from build123d import *
from OCP.BRepFilletAPI import BRepFilletAPI_MakeChamfer
from build123d.topology import SkipClean

# Parameters (mm, degrees)
SKETCH1_R                 = 12
SKETCH1_R_2               = 8
BOSS_EXTRUDE4_DEPTH       = 2
BOSS_EXTRUDE5_START       = 2
SKETCH1_9_R               = 12
SKETCH1_9_R_2             = 9
BOSS_EXTRUDE5_DEPTH       = 4
BOSS_EXTRUDE6_START       = 2
BOSS_EXTRUDE6_DEPTH       = 2
BOSS_EXTRUDE7_START       = 4
BOSS_EXTRUDE7_DEPTH       = 2
SKETCH1_12_W              = 60
SKETCH1_12_H              = 60
SKETCH1_12_R              = 12
SKETCH1_12_R_2            = 9
SKETCH1_12_R_3            = 8
BOSS_EXTRUDE8_DEPTH       = 2
BOSS_EXTRUDE9_DEPTH       = 6
CHAMFER1_SIZE             = 1
CHAMFER1_SIZE2            = 0.176326981
BOSS_EXTRUDE10_DEPTH      = 6
BOSS_EXTRUDE11_DEPTH      = 20
BOSS_EXTRUDE12_DEPTH      = 2
BOSS_EXTRUDE12_DEPTH_BACK = 2
SKETCH1_14_R              = 8
CUT_EXTRUDE1_DEPTH        = 47.904157598


with BuildPart() as part:
    # Sketch1 → Boss-Extrude4 (new body)
    with BuildSketch(Plane(origin=(0, 0, 0), x_dir=(1, 0, 0), z_dir=(0, 1, 0))):
        with Locations(Location((0, 0, 0), (0, 0, 270))):
            Circle(SKETCH1_R)
        with Locations(Location((0, 0, 0), (0, 0, 270))):
            Circle(SKETCH1_R_2, mode=Mode.SUBTRACT)
    extrude(amount=BOSS_EXTRUDE4_DEPTH)

    # Sketch1<9> → Boss-Extrude5 (add)
    with BuildSketch(Plane(origin=(0, 0, 0), x_dir=(1, 0, 0), z_dir=(0, 1, 0)).offset(BOSS_EXTRUDE5_START)):
        with Locations(Location((0, 0, 0), (0, 0, 270))):
            Circle(SKETCH1_9_R)
        with Locations(Location((0, 0, 0), (0, 0, 270))):
            Circle(SKETCH1_9_R_2, mode=Mode.SUBTRACT)
    extrude(amount=BOSS_EXTRUDE5_DEPTH)

    # Sketch1<10> → Boss-Extrude6 (add)
    with SkipClean():  # the faces are left unmerged after this step: merging them gives an invalid solid
        with BuildSketch(Plane(origin=(0, 0, 0), x_dir=(1, 0, 0), z_dir=(0, 1, 0)).offset(BOSS_EXTRUDE6_START)):
            with BuildLine():
                ThreePointArc((0, 8), (2.070552361, 7.72740661), (4, 6.92820323))
                Line((4, 6.92820323), (4.5, 7.794228634))
                ThreePointArc((4.5, 7.794228634), (2.329371406, 8.693332437), (0, 9))
                Line((0, 9), (0, 8))
            make_face()
            with BuildLine():
                ThreePointArc((-8, 0), (-7.72740661, 2.070552361), (-6.92820323, 4))
                Line((-6.92820323, 4), (-7.794228634, 4.5))
                ThreePointArc((-7.794228634, 4.5), (-8.693332437, 2.329371406), (-9, 0))
                Line((-9, 0), (-8, 0))
            make_face()
            with BuildLine():
                Line((0, -9), (0, -8))
                ThreePointArc((0, -8), (-2.070552361, -7.72740661), (-4, -6.92820323))
                Line((-4, -6.92820323), (-4.5, -7.794228634))
                ThreePointArc((-4.5, -7.794228634), (-2.329371406, -8.693332437), (0, -9))
            make_face()
            with BuildLine():
                Line((9, 0), (8, 0))
                ThreePointArc((8, 0), (7.72740661, -2.070552361), (6.92820323, -4))
                Line((6.92820323, -4), (7.794228634, -4.5))
                ThreePointArc((7.794228634, -4.5), (8.693332437, -2.329371406), (9, 0))
            make_face()
        extrude(amount=BOSS_EXTRUDE6_DEPTH)

    # Sketch1<11> → Boss-Extrude7 (add)
    with SkipClean():  # the faces are left unmerged after this step: merging them gives an invalid solid
        with BuildSketch(Plane(origin=(0, 0, 0), x_dir=(1, 0, 0), z_dir=(0, 1, 0)).offset(BOSS_EXTRUDE7_START)):
            with BuildLine():
                ThreePointArc((0, 8), (2.070552361, 7.72740661), (4, 6.92820323))
                Line((4, 6.92820323), (4.5, 7.794228634))
                ThreePointArc((4.5, 7.794228634), (2.329371406, 8.693332437), (0, 9))
                Line((0, 9), (0, 8))
            make_face()
            with BuildLine():
                ThreePointArc((4, 6.92820323), (5.656854249, 5.656854249), (6.92820323, 4))
                Line((6.92820323, 4), (7.794228634, 4.5))
                ThreePointArc((7.794228634, 4.5), (6.363961031, 6.363961031), (4.5, 7.794228634))
                Line((4.5, 7.794228634), (4, 6.92820323))
            make_face()
            with BuildLine():
                ThreePointArc((-8, 0), (-7.72740661, 2.070552361), (-6.92820323, 4))
                Line((-6.92820323, 4), (-7.794228634, 4.5))
                ThreePointArc((-7.794228634, 4.5), (-8.693332437, 2.329371406), (-9, 0))
                Line((-9, 0), (-8, 0))
            make_face()
            with BuildLine():
                ThreePointArc((-6.92820323, 4), (-5.656854249, 5.656854249), (-4, 6.92820323))
                Line((-4, 6.92820323), (-4.5, 7.794228634))
                ThreePointArc((-4.5, 7.794228634), (-6.363961031, 6.363961031), (-7.794228634, 4.5))
                Line((-7.794228634, 4.5), (-6.92820323, 4))
            make_face()
            with BuildLine():
                Line((-4.5, -7.794228634), (-4, -6.92820323))
                ThreePointArc((-4, -6.92820323), (-5.656854249, -5.656854249), (-6.92820323, -4))
                Line((-6.92820323, -4), (-7.794228634, -4.5))
                ThreePointArc((-7.794228634, -4.5), (-6.363961031, -6.363961031), (-4.5, -7.794228634))
            make_face()
            with BuildLine():
                Line((0, -9), (0, -8))
                ThreePointArc((0, -8), (-2.070552361, -7.72740661), (-4, -6.92820323))
                Line((-4, -6.92820323), (-4.5, -7.794228634))
                ThreePointArc((-4.5, -7.794228634), (-2.329371406, -8.693332437), (0, -9))
            make_face()
            with BuildLine():
                Line((9, 0), (8, 0))
                ThreePointArc((8, 0), (7.72740661, -2.070552361), (6.92820323, -4))
                Line((6.92820323, -4), (7.794228634, -4.5))
                ThreePointArc((7.794228634, -4.5), (8.693332437, -2.329371406), (9, 0))
            make_face()
            with BuildLine():
                Line((7.794228634, -4.5), (6.92820323, -4))
                ThreePointArc((6.92820323, -4), (5.656854249, -5.656854249), (4, -6.92820323))
                Line((4, -6.92820323), (4.5, -7.794228634))
                ThreePointArc((4.5, -7.794228634), (6.363961031, -6.363961031), (7.794228634, -4.5))
            make_face()
        extrude(amount=BOSS_EXTRUDE7_DEPTH)

    # Sketch1<12> → Boss-Extrude8 (add)
    # profile 1 of 2: a face of its own
    with BuildSketch(Plane(origin=(0, 0, 0), x_dir=(1, 0, 0), z_dir=(0, 1, 0))):
        Rectangle(SKETCH1_12_W, SKETCH1_12_H)
        with Locations(Location((0, 0, 0), (0, 0, 270))):
            Circle(SKETCH1_12_R, mode=Mode.SUBTRACT)
    # profile 2 of 2: a face of its own
    with BuildSketch(Plane(origin=(0, 0, 0), x_dir=(1, 0, 0), z_dir=(0, 1, 0))):
        Circle(SKETCH1_12_R_2)
        with Locations(Location((0, 0, 0), (0, 0, 270))):
            Circle(SKETCH1_12_R_3, mode=Mode.SUBTRACT)
    extrude(amount=BOSS_EXTRUDE8_DEPTH)

    # Sketch3 → Boss-Extrude9 (add)
    with BuildSketch(Plane.XZ):
        Polygon((-30, -30), (30, -30), (30, -28), (-28, -28), (-28, 30), (-30, 30), align=None)
        Polygon((30, -26), (30, -24), (-24, -24), (-24, 30), (-26, 30), (-26, -26), align=None)
    extrude(amount=BOSS_EXTRUDE9_DEPTH)

    # Chamfer1: one chamfer whose edges measure the first distance from different faces: ONE call of the kernel's chamfer builder (chamfer() names one face for all edges)
    chamfer1_edges_1 = [part.edges().sort_by_distance(p)[0] for p in [
        (-28, -6, 1),
    ]]
    chamfer1_side_1 = [part.faces().sort_by_distance(p)[0] for p in [
        (-28, -3, 1),
    ]]
    chamfer1_edges_2 = [part.edges().sort_by_distance(p)[0] for p in [
        (1, -6, -28),
    ]]
    chamfer1_side_2 = [part.faces().sort_by_distance(p)[0] for p in [
        (1, -3, -28),
    ]]
    chamfer1_edges_3 = [part.edges().sort_by_distance(p)[0] for p in [
        (-29, -6, 30),
    ]]
    chamfer1_side_3 = [part.faces().sort_by_distance(p)[0] for p in [
        (-4.5, 0.333333333, 30),
    ]]
    chamfer1_edges_4 = [part.edges().sort_by_distance(p)[0] for p in [
        (-30, -6, 0),
    ]]
    chamfer1_side_4 = [part.faces().sort_by_distance(p)[0] for p in [
        (-30, -2, 0),
    ]]
    chamfer1_edges_5 = [part.edges().sort_by_distance(p)[0] for p in [
        (0, -6, -30),
    ]]
    chamfer1_side_5 = [part.faces().sort_by_distance(p)[0] for p in [
        (0, -2, -30),
    ]]
    chamfer1_edges_6 = [part.edges().sort_by_distance(p)[0] for p in [
        (30, -6, -29),
    ]]
    chamfer1_side_6 = [part.faces().sort_by_distance(p)[0] for p in [
        (30, 0.333333333, -4.5),
    ]]
    chamfer1 = BRepFilletAPI_MakeChamfer(part.part.solid().wrapped)
    for e in chamfer1_edges_1:
        chamfer1.Add(CHAMFER1_SIZE, CHAMFER1_SIZE2, e.wrapped, chamfer1_side_1[0].wrapped)  # the first distance lies on this face
    for e in chamfer1_edges_2:
        chamfer1.Add(CHAMFER1_SIZE, CHAMFER1_SIZE2, e.wrapped, chamfer1_side_2[0].wrapped)  # the first distance lies on this face
    for e in chamfer1_edges_3:
        chamfer1.Add(CHAMFER1_SIZE, CHAMFER1_SIZE2, e.wrapped, chamfer1_side_3[0].wrapped)  # the first distance lies on this face
    for e in chamfer1_edges_4:
        chamfer1.Add(CHAMFER1_SIZE, CHAMFER1_SIZE2, e.wrapped, chamfer1_side_4[0].wrapped)  # the first distance lies on this face
    for e in chamfer1_edges_5:
        chamfer1.Add(CHAMFER1_SIZE, CHAMFER1_SIZE2, e.wrapped, chamfer1_side_5[0].wrapped)  # the first distance lies on this face
    for e in chamfer1_edges_6:
        chamfer1.Add(CHAMFER1_SIZE, CHAMFER1_SIZE2, e.wrapped, chamfer1_side_6[0].wrapped)  # the first distance lies on this face
    add(Compound.cast(chamfer1.Shape()), mode=Mode.REPLACE)

    # Sketch6 → Boss-Extrude10 (add)
    with BuildSketch(Plane.XZ):
        Polygon((-24, 30), (-24, 28), (28, 28), (28, -24), (30, -24), (30, 30), align=None)
    extrude(amount=BOSS_EXTRUDE10_DEPTH)

    # Sketch3<3> → Boss-Extrude11 (add)
    with SkipClean():  # the faces are left unmerged after this step: merging them gives an invalid solid
        with BuildSketch(Plane.XZ):
            Polygon((-26, 30), (-26, -26), (-24, -24), (-24, 30), align=None)
            Polygon((-26, -26), (30, -26), (30, -24), (-24, -24), align=None)
        extrude(amount=BOSS_EXTRUDE11_DEPTH)

    # Sketch9 → Boss-Extrude12 (add, two sides: drawn at the far end of the back side and taken through both)
    with SkipClean():  # the faces are left unmerged after this step: merging them gives an invalid solid
        with BuildSketch(Plane(origin=(0, 0, 0), x_dir=(-0.7071067811865472, 0, -0.7071067811865478), z_dir=(0.7071067811865478, 0, -0.7071067811865472)).offset(-BOSS_EXTRUDE12_DEPTH_BACK)):
            Polygon((33.941125497, -20), (33.941125497, 0), (8, 0), (8, -4.714045208), align=None)
            Polygon((8, -4.714045208), (8, 0), (0, 0), align=None)
        extrude(amount=BOSS_EXTRUDE12_DEPTH + BOSS_EXTRUDE12_DEPTH_BACK)

    # Sketch1<14> → Cut-Extrude1 (cut, through all)
    with SkipClean():  # the faces are left unmerged after this step: merging them gives an invalid solid
        with BuildSketch(Plane(origin=(0, 0, 0), x_dir=(1, 0, 0), z_dir=(0, 1, 0))):
            with Locations(Location((0, 0, 0), (0, 0, 90))):
                Circle(SKETCH1_14_R)
        extrude(amount=-CUT_EXTRUDE1_DEPTH, mode=Mode.SUBTRACT)


solid = part.part
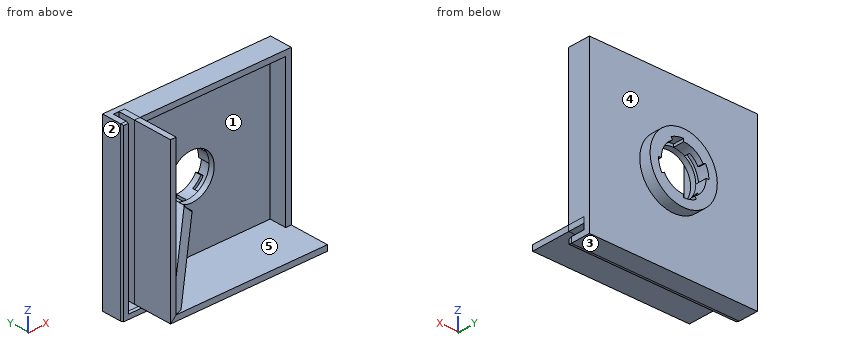
Check sheet for the modelled part. Datum: model origin and axes. Units: mm. Face numbers are marked on the shaded views. A direction names the side the tool comes from. Give positions to 0.01 mm unless a question says otherwise; leave off trailing zeros. Loops run counter-clockwise (first coordinate to the right, second up) from the corner with the lowest first, then second, coordinate; pieces in that order, holes last. Notation, with made-up numbers: M 72,88.25 L 116,88.25 A20 ccw 116,108.25 Z; hole C -4,-20.75 d4. An arc over 180 degrees is marked long. Return JSON: item names as keys, results as strings. Group by question number.
1. Mould release check, pull along Z, two halves, no side actions. Record for the marked faces 1, 2 and 3: released by +Z, released by -Z, zero draft, split by the parting line, or undercut.
2. Thickness scan on L1, parallel to X at y = -1.75, z = 16; L2, parallel to X at y = 0.75, z = 0. Record the ranges inside material, lowest first.
3. Cross-section at C-C on y = 3. Record the boundary of the cut face in (x, z), plus the area to 3 significant figures.
4. Tool access check on the marked faces 4 and 5. Record the directions out of +Z, -Z, +X, -X, +Y, -Y that give a thin tool (end or side, any length) a straight path to the whole face; none if there is none.
5. Cross-section at A-A on y = -2. Record the boundary of the cut face in (x, z).
6. Cross-section at B-B on z = 3. Record the boundary of the cut face in (x, y).
7. Go/stop test with flat-tipped pins: pin 1 (15.5 mm diameter, centred on x = 2, z = 10.5, fed in from -Y); pin 2 (6 mm diameter, centred on y = -16, z = -16.5, fed in from +X); pin 3 (7 mm diameter, centred on y = -13, z = 7.5, fed in from -X); pin 4 (2.5 mm diameter, centred on x = 5.5, z = -2.5, fed in from +Y). Record where each tip stops, or that it passes through.
Return value:
{
 "1": {"face 1": "undercut", "face 2": "zero draft", "face 3": "released by -Z"},
 "2": {"L1": "-30 to -28, -26 to -24, 28 to 30", "L2": "-30 to -8, 8 to 30"},
 "3": {"outline": "C 0,0 d24; hole M -9,0 L -8,0 A8 ccw -6.93,-4 L -7.79,-4.5 A9 ccw 0,-9 L 0,-8 A8 ccw 4,-6.93 L 4.5,-7.79 A9 ccw 9,0 L 8,0 A8 ccw 6.93,4 L 7.79,4.5 A9 ccw 0,9 L 0,8 A8 ccw -4,6.93 L -4.5,7.79 A9 ccw Z", "area": "216 mm^2"},
 "4": {"face 4": "+Y", "face 5": "-Y"},
 "5": {"outline": "M -30,-30 L 30,-30 L 30,-28 L -28,-28 L -28,30 L -30,30 Z; M -26,-26 L 30,-26 L 30,30 L -26,30 Z; hole M -24,-21.17 L -6.89,-4.06 A8 ccw -4.06,-6.89 L -21.17,-24 L 28,-24 L 28,28 L -24,28 Z"},
 "6": {"outline": "M -30,-5 L -29.82,-6 L -28.18,-6 L -28,-5 L -28,0 L -26,0 L -26,-20 L -24,-20 L -24,0 L -7.42,0 L -7.42,2 L -8.49,2 L -8.49,6 L -11.62,6 L -11.62,2 L -30,2 Z; M 7.42,0 L 28,0 L 28,-6 L 30,-6 L 30,2 L 11.62,2 L 11.62,6 L 7.42,6 Z"},
 "7": {"pin 1": "y = 0", "pin 2": "x = -14.25", "pin 3": "x = -26", "pin 4": "through"}
}
